Read the model definition and answer for the solid it produces. Units are mm, in the model's axes. A direction names the side the tool comes from. Coordinates: 2 decimals unless noted, no trailing zeros. Order: outer loops, then holes, each group sorted by start corner. A loop starts at its lowest first (then second) coordinate and runs counter-clockwise, first axis right, second up. Notation, with made-up numbers: (-27, 57.25) - (-11, 57.25) arc R16 cw to (-11, 76.25) - close; hole circle Ø7 at (-7.5, -20.75). An arc over 180 degrees is marked (long way). Write item = value, one per line.
from build123d import *

# Parameters (mm, degrees)
F0_R     = 3.175
F0_R_2   = 1.5875
F1_DEPTH = 3.048


with BuildPart() as f1:
    # F0 (on Front) → F1 (new body)
    with BuildSketch(Plane.XZ):
        with BuildLine():
            ThreePointArc((-9.464408, 69.282927), (-0.537188, 58.700422), (9.525, 68.210262))
            ThreePointArc((9.525, 68.210262), (9.50984, 68.74745), (9.464408, 69.282927))
            ThreePointArc((9.464408, 69.282927), (0, 77.735262), (-9.464408, 69.282927))
        make_face()
        with Locations((0, 68.210262)):
            Circle(F0_R, mode=Mode.SUBTRACT)
        with BuildLine():
            ThreePointArc((9.464408, 69.282927), (9.50984, 68.74745), (9.525, 68.210262))
            ThreePointArc((9.525, 68.210262), (-0.537188, 58.700422), (-9.464408, 69.282927))
            Line((-9.464408, 69.282927), (-15.750459, 19.394869))
            ThreePointArc((-15.750459, 19.394869), (0, 33.285262), (15.750459, 19.394869))
            Line((15.750459, 19.394869), (9.464408, 69.282927))
        make_face()
        with Locations((-4.10057, 53.704553)):
            Circle(F0_R_2, mode=Mode.SUBTRACT)
        with BuildLine():
            ThreePointArc((15.875, 17.410262), (15.843834, 18.404518), (15.750459, 19.394869))
            ThreePointArc((15.750459, 19.394869), (0, 33.285262), (-15.750459, 19.394869))
            ThreePointArc((-15.750459, 19.394869), (-15.873818, 17.603994), (-15.794203, 15.810642))
            ThreePointArc((-15.794203, 15.810642), (-0.113839, 1.53567), (15.769637, 15.584293))
            Line((15.769637, 15.584293), (15.815592, 16.038155))
            ThreePointArc((15.815592, 16.038155), (15.860141, 16.723566), (15.875, 17.410262))
        make_face()
        with Locations((0, 17.410262)):
            Circle(F0_R_2, mode=Mode.SUBTRACT)
        with BuildLine():
            ThreePointArc((15.769637, 15.584293), (-0.113839, 1.53567), (-15.794203, 15.810642))
            Line((-15.794203, 15.810642), (-9.525, -46.089738))
            ThreePointArc((-9.525, -46.089738), (0, -36.564738), (9.525, -46.089738))
            ThreePointArc((9.525, -46.089738), (6.970557, -52.581037), (0.677344, -55.590624))
            Line((0.677344, -55.590624), (44.732405, -54.022212))
            ThreePointArc((44.732405, -54.022212), (36.513756, -46.230963), (44.45, -38.152238))
            Line((44.45, -38.152238), (18.932522, -37.240899))
            ThreePointArc((18.932522, -37.240899), (13.224065, -34.520616), (11.306519, -28.494884))
            Line((11.306519, -28.494884), (15.769637, 15.584293))
        make_face()
        with BuildLine():
            ThreePointArc((15.769637, 15.584293), (15.794245, 15.811059), (15.815592, 16.038155))
            Line((15.815592, 16.038155), (15.769637, 15.584293))
        make_face()
        with BuildLine():
            ThreePointArc((9.525, -46.089738), (0, -36.564738), (-9.525, -46.089738))
            ThreePointArc((-9.525, -46.089738), (-6.735192, -52.82493), (0, -55.614738))
            Line((0, -55.614738), (0.677344, -55.590624))
            ThreePointArc((0.677344, -55.590624), (6.970557, -52.581037), (9.525, -46.089738))
        make_face()
        with Locations((0, -46.089738)):
            Circle(F0_R_2, mode=Mode.SUBTRACT)
        with BuildLine():
            Line((0.677344, -55.590624), (0, -55.614738))
            ThreePointArc((0, -55.614738), (0.338886, -55.608707), (0.677344, -55.590624))
        make_face()
        with BuildLine():
            ThreePointArc((52.3875, -46.089738), (50.06266, -40.477078), (44.45, -38.152238))
            ThreePointArc((44.45, -38.152238), (36.513756, -46.230963), (44.732405, -54.022212))
            ThreePointArc((44.732405, -54.022212), (50.161633, -51.601648), (52.3875, -46.089738))
        make_face()
        with Locations((44.45, -46.089738)):
            Circle(F0_R_2, mode=Mode.SUBTRACT)
    extrude(amount=F1_DEPTH)


solid = f1.part
1) For faces 1 (the face through (-6.81, -1.5, -52.75)), 2 (the face through (13.284, -1.503, -34.589)), determine the directions among +Z, -Z, +X, -X, +Y, -Y from which every point of the face is accessible in a straight line to the end or side of a thin tool.
Returned:
face_1 = -Z, -X, +Y, -Y
face_2 = +X, +Y, -Y
2) The part is cut by section A-A (y = -1.9). Count the separate pieces of the cut face and the enclosed holes in it, and give its area (3 significant figures).
Returned:
separate_pieces = 1
enclosed_holes = 5
area = 3,870 mm^2
3) Determine the mould class of faces 3 (the face through (3, 0, -3)), 4 (the face through (0.194, -1.503, 77.733)), 5 (the face through (-4.31, -1.5, 55.28)) for opening direction X: pulls with the +X half, pulls with the -X half, needs draft (parallel to the pull), parting line crosses it, or undercut.
Returned:
face_3 = needs draft
face_4 = parting line crosses it
face_5 = undercut
4) The part is cut by section C-C (x = 40). Determine the outline of the cut face in (y, z), and give its area (3 significant figures).
Returned:
outline = (-3.05, -54.19) - (0, -54.19) - (0, -37.99) - (-3.05, -37.99) - close
area = 49.4 mm^2
5) Straight lines are drawn through the part: line 1 along Z through (x, y) = (0.5, -2); line 2 along X through (y, z) = (-1.65, 53.5); line 3 along X through (y, z) = (-0.8, 53). For each, find the intervals that lie inside material, in ascending order. Write a range as from..to.
Returned:
line_1 = -55.6..-47.6, -44.58..15.9, 18.92..65.07, 71.35..77.72
line_2 = -11.45..-5.67, -2.53..11.45
line_3 = -11.52..-5.52, -2.68..11.52
6) A flat-ended cylindrical pin translates along its axis: pin 1 Ø1 at (x, y) = (28, -1.5) entering from -Z. Find the tip coordinate at first contact, or state that the pin passes through.
Returned:
pin_1 = -54.64
7) The part is cut by section B-B (z = 38). Determine the outline of the cut face in (x, y), and give its area (3 significant figures).
Returned:
outline = (-13.41, -3.05) - (13.41, -3.05) - (13.41, 0) - (-13.41, 0) - close
area = 81.7 mm^2
